```python
from build123d import *

# Parameters (mm, degrees)
SM_BASE_FLANGE_1_DEPTH = 180
CUT_EXTRUDE_1_DEPTH    = 184.524521522


# Sheet-metal steps are written as plain solids
with BuildPart() as part:
    # Sketch 1 → Базовая кромка1 (new body)
    with BuildSketch(Plane.XY):
        with BuildLine():
            Line((0, 0), (3.2, 0))
            ThreePointArc((3.2, 0), (3.765685425, -0.234314575), (4, -0.8))
            Line((4, -0.8), (4, -5.9))
            ThreePointArc((4, -5.9), (4.46862915, -7.03137085), (5.6, -7.5))
            Line((5.6, -7.5), (29.4, -7.5))
            ThreePointArc((29.4, -7.5), (30.53137085, -7.03137085), (31, -5.9))
            Line((31, -5.9), (31, -0.8))
            ThreePointArc((31, -0.8), (31.234314575, -0.234314575), (31.8, 0))
            Line((31.8, 0), (35, 0))
            Line((35, 0), (35, 0.8))
            Line((35, 0.8), (31.8, 0.8))
            ThreePointArc((31.8, 0.8), (30.66862915, 0.33137085), (30.2, -0.8))
            Line((30.2, -0.8), (30.2, -5.9))
            ThreePointArc((30.2, -5.9), (29.965685425, -6.465685425), (29.4, -6.7))
            Line((29.4, -6.7), (5.6, -6.7))
            ThreePointArc((5.6, -6.7), (5.034314575, -6.465685425), (4.8, -5.9))
            Line((4.8, -5.9), (4.8, -0.8))
            ThreePointArc((4.8, -0.8), (4.33137085, 0.33137085), (3.2, 0.8))
            Line((3.2, 0.8), (0, 0.8))
            Line((0, 0.8), (0, 0))
        make_face()
    extrude(amount=SM_BASE_FLANGE_1_DEPTH)

    # Эскиз6 → Вырез-Вытянуть1 (cut, through all)
    with BuildSketch(Plane(origin=(0, -6.7, 0), x_dir=(1, 0, 0), z_dir=(0, 1, 0))):
        with BuildLine():
            Line((20.6, -6), (20.6, -16))
            ThreePointArc((20.6, -16), (17.5, -19.1), (14.4, -16))
            Line((14.4, -16), (14.4, -6))
            ThreePointArc((14.4, -6), (17.5, -2.9), (20.6, -6))
        make_face()
        with BuildLine():
            Line((20.6, -30), (20.6, -40))
            ThreePointArc((20.6, -40), (17.5, -43.1), (14.4, -40))
            Line((14.4, -40), (14.4, -30))
            ThreePointArc((14.4, -30), (17.5, -26.9), (20.6, -30))
        make_face()
        with BuildLine():
            Line((20.6, -54), (20.6, -64))
            ThreePointArc((20.6, -64), (17.5, -67.1), (14.4, -64))
            Line((14.4, -64), (14.4, -54))
            ThreePointArc((14.4, -54), (17.5, -50.9), (20.6, -54))
        make_face()
        with BuildLine():
            Line((20.6, -78), (20.6, -88))
            ThreePointArc((20.6, -88), (17.5, -91.1), (14.4, -88))
            Line((14.4, -88), (14.4, -78))
            ThreePointArc((14.4, -78), (17.5, -74.9), (20.6, -78))
        make_face()
        with BuildLine():
            Line((20.6, -102), (20.6, -112))
            ThreePointArc((20.6, -112), (17.5, -115.1), (14.4, -112))
            Line((14.4, -112), (14.4, -102))
            ThreePointArc((14.4, -102), (17.5, -98.9), (20.6, -102))
        make_face()
        with BuildLine():
            Line((20.6, -126), (20.6, -136))
            ThreePointArc((20.6, -136), (17.5, -139.1), (14.4, -136))
            Line((14.4, -136), (14.4, -126))
            ThreePointArc((14.4, -126), (17.5, -122.9), (20.6, -126))
        make_face()
        with BuildLine():
            Line((20.6, -150), (20.6, -160))
            ThreePointArc((20.6, -160), (17.5, -163.1), (14.4, -160))
            Line((14.4, -160), (14.4, -150))
            ThreePointArc((14.4, -150), (17.5, -146.9), (20.6, -150))
        make_face()
        with BuildLine():
            Line((20.6, -174), (20.6, -184))
            ThreePointArc((20.6, -184), (17.5, -187.1), (14.4, -184))
            Line((14.4, -184), (14.4, -174))
            ThreePointArc((14.4, -174), (17.5, -170.9), (20.6, -174))
        make_face()
    extrude(amount=-CUT_EXTRUDE_1_DEPTH, mode=Mode.SUBTRACT)


solid = part.part
```
Can you work these out from the model? Positions are in its coordinate system, mm. A direction names the side the tool comes from. Give positions to 0.01 mm unless a question says otherwise; leave off trailing zeros. Order: outer loops, then holes, each group sorted by start corner. A loop starts at its lowest first (then second) coordinate and runs counter-clockwise, first axis right, second up. Notation, with made-up numbers: (14.25, -38) - (52.25, -38) arc R25 cw to (52.25, -8) - close; hole circle Ø2 at (3.5, 83.25). An arc over 180 degrees is marked (long way). Use a Markdown table: item, result. Add a question column.
Q1. I'm going to push flat-ended pins straight in: pin 1 (0.9 mm diameter, centred on y = -7, z = 157, fed in from -X); pin 2 (2.5 mm diameter, centred on x = 1.5, z = 80.5, fed in from -Y); pin 3 (0.6 mm diameter, centred on y = -7, z = 129.5, fed in from -X). Where does each tip first touch, or does it pass through?
Q2. If we section it at B-B on y = -2.75: Write out the boundary of the cut face in (x, z).
Q3. If we section it at C-C on z = 69: Write out the boundary of the cut face in (x, y).
Q4. If we mould it in two halves opening along Z, with no side actions, what happens to faces 5 (the flat face through (30.4, -4.6, 180)), 6 (the cylindrical face through (17.4, -7.1, 146.9)), 7 (the flat face through (4, -3, 89))? For each: released by +Z, released by -Z, zero draft, split by the parting line, or undercut.
Q5. Please list where these lines run through material, in increasing order: line 1 along X through (y, z) = (-5, 111); line 2 along Y through (x, z) = (11, 37); line 3 along Y through (x, z) = (2, 81.5).
Q6. If we section it at D-D on x = 25.5: Write out the boundary of the cut face in (y, z), plus the area to 3 significant figures.
Q7. If we section it at A-A on x = 17.5: Count the separate pieces of the cut face and the enclosed holes in it, plus the area to 3 significant figures.
Q8. On a 3-axis mill with a long thin cutter (end or side, diameter ignored), from which of +Z, -Z, +X, -X, +Y, -Y can I reach the whole of each face in a straight line? I mean faces 1 (the flat face through (23, -6.7, 89)), 2 (the flat face through (33, 0, 89)), 3 (the cylindrical face through (17.4, -7.1, 170.9)), 4 (the cylindrical face through (17.6, -7.1, 163.1)). Say none if no direction works.
Answers follow:
| question | item | result |
|---|---|---|
| 1 | pin 1 | stops at x = 4.14 |
| 1 | pin 2 | stops at y = 0 |
| 1 | pin 3 | stops at x = 4.21 |
| 2 | outline | (4, 0) - (4.8, 0) - (4.8, 180) - (4, 180) - close; (30.2, 0) - (31, 0) - (31, 180) - (30.2, 180) - close |
| 3 | outline | (0, 0) - (3.2, 0) arc R0.8 cw to (4, -0.8) - (4, -5.9) arc R1.6 ccw to (5.6, -7.5) - (29.4, -7.5) arc R1.6 ccw to (31, -5.9) - (31, -0.8) arc R0.8 cw to (31.8, 0) - (35, 0) - (35, 0.8) - (31.8, 0.8) arc R1.6 ccw to (30.2, -0.8) - (30.2, -5.9) arc R0.8 cw to (29.4, -6.7) - (5.6, -6.7) arc R0.8 cw to (4.8, -5.9) - (4.8, -0.8) arc R1.6 ccw to (3.2, 0.8) - (0, 0.8) - close |
| 4 | face 5 | released by +Z |
| 4 | face 6 | undercut |
| 4 | face 7 | zero draft |
| 5 | line 1 | x = 4 to 4.8, 30.2 to 31 |
| 5 | line 2 | y = -7.5 to -6.7 |
| 5 | line 3 | y = 0 to 0.8 |
| 6 | outline | (-7.5, 0) - (-6.7, 0) - (-6.7, 180) - (-7.5, 180) - close |
| 6 | area | 144 mm^2 |
| 7 | separate pieces | 8 |
| 7 | enclosed holes | 0 |
| 7 | area | 46.0 mm^2 |
| 8 | face 1 | +Z, -Z, +Y |
| 8 | face 2 | +Z, -Z, +X, -Y |
| 8 | face 3 | +Z, +Y, -Y |
| 8 | face 4 | +Y, -Y |
